```python
from build123d import *

# Parameters (mm, degrees)
F0_W     = 26.5914327465
F0_H     = 12.9917515442
F2_W     = 3
F2_H     = 11
F3_DEPTH = 25
F5_D     = 5
F7_D     = 2.4
F7_DEPTH = 32.7668578753


with BuildPart() as f1:
    # F0 (on Front) → F1 (revolve)
    with BuildSketch(Plane.XZ):
        with Locations((19.4701415021, 6.4958757721)):
            Rectangle(F0_W, F0_H)
    revolve(axis=Axis((0, 0, 8.0647598952), (0, 0, -1)))

    # F2 (on face) → F3 (cut)
    with BuildSketch(Plane.XY.offset(12.9917515442)):
        Polygon((-5.7890059302, -2.1473090164), (-6.0011490459, 1.4524929605), (-35.6950574279, 1.4524929605), (-35.6950574279, -2.1473090164), align=None)
        with Locations((23.4585951418, 0.467357954)):
            Rectangle(F2_W, F2_H)
    extrude(amount=-F3_DEPTH, mode=Mode.SUBTRACT)

    # F5 (through all)
    with Locations(Plane.XY.offset(12.9917515442)):
        with Locations((-10.3396493942, 10.5901481584), (6.8767020359, 13.1061266864), (14.5896849828, -2.4901164053), (2.1402191687, -14.6451032608), (-13.2669567932, -6.5610551786), (-4.8388554715, 20.6837356091), (18.1761129583, 10.9936508379), (-8.2428784436, -19.577701499), (16.0723110631, -13.8892857308), (10.152108036, 19.7349414229), (10.152108036, -19.7349414229), (-16.224399209, -14.8012051359)):
            Hole(F5_D / 2)

    # F7 (through all, one way)
    with BuildSketch(Plane.XZ):
        with Locations((-17.7818648517, 6.34881109)):
            Circle(F7_D / 2)
    extrude(amount=-F7_DEPTH, mode=Mode.SUBTRACT)


solid = f1.part
```
Read the model definition and answer for the solid it produces. Units are mm, in the model's axes. A direction names the side the tool comes from. Give positions to 0.01 mm unless a question says otherwise; leave off trailing zeros. Write each loop counter-clockwise with the first axis right and the second up, starting at its lowest first coordinate (ties: lowest second). Pieces come first, ordered by that corner, then holes. Notation, with made-up numbers: M -25,-11.75 L 13,-11.75 A20 ccw 13,-3.75 Z; hole C 78,36.25 d1. An arc over 180 degrees is marked long. Put each result on its own line as item: value. Start each with the question number.
1. Each of these flat-tipped pins is pushed along its axis until it touches: pin 1 Ø4 at (x, z) = (-23.5, 4.5) entering from +Y; pin 2 Ø5 at (x, z) = (2.5, 2) entering from -Y; pin 3 Ø3.5 at (x, z) = (23, 7) entering from +Y. Where does it stop, or does it pass through?
2. Which of the six approach directions +Z, -Z, +X, -X, +Y, -Y give full straight-line access (tool end or side, diameter ignored) to faces 5 (the flat face through (21.959, 0, 7)), 6 (the flat face through (0, 7, 0)), 7 (the flat face through (-19, -2.147, 7))?
3. The part is cut by section C-C, the plane y = 24. Give the vertices of the cut face in (x, z), and give its area (3 significant figures).
4. The part is cut by section A-A, the plane x = 3.5. Give the vertices of the cut face in (y, z), and give its area (3 significant figures).
5. Consider line 1 along X through (y, z) = (-4, 9.75); line 2 along X through (y, z) = (18.5, 3.5); line 3 along Y through (x, z) = (3.5, 9.5). Determine where each line is inside the solid, lowest interval first.
6. For a pull along Y with two mould halves and no side action, classify faces 1 (the cylindrical face through (26.435, -19.359, 6.587)), 2 (the cylindrical face through (17.087, -2.38, 6.405)), 3 (the cylindrical face through (-18.734, 14.669, 5.619)), 4 (the cylindrical face through (2.682, -17.086, 6.405)) as released by +Y, released by -Y, zero draft, split by the parting line, or undercut.
7. The part is cut by section B-B, the plane z = 2.5. Give the number of separate pieces and of enclosed holes in the cut face, and give its area (3 significant figures).
Final values:
1. pin 1: stops at y = 24.73
1. pin 2: stops at y = -32.77
1. pin 3: stops at y = 24.94
2. face 5: +Z, -Z
2. face 6: -Z, +X, -X, +Y, -Y
2. face 7: +Z, -Z, -X
3. outline: M -22.31,0 L 22.31,0 L 22.31,12.99 L -22.31,12.99 Z; hole C -17.78,6.35 d2.4
3. area: 575 mm²
4. outline: M -32.58,0 L -16.74,0 L -16.74,12.99 L -32.58,12.99 Z; M -12.55,0 L -5.09,0 L -5.09,12.99 L -12.55,12.99 Z; M 5.09,0 L 32.58,0 L 32.58,12.99 L 5.09,12.99 Z
4. area: 660 mm²
5. line 1: x = -32.52 to -4.7, 4.7 to 12.6, 16.58 to 21.96, 24.96 to 32.52
5. line 2: x = -27.04 to -6.06, -3.62 to 7.98, 12.33 to 27.04
5. line 3: y = -32.58 to -16.74, -12.55 to -5.09, 5.09 to 32.58
6. face 1: split by the parting line
6. face 2: undercut
6. face 3: zero draft
6. face 4: undercut
7. separate pieces: 1
7. enclosed holes: 13
7. area: 2,890 mm²
